Could you check a few things on this model? Use its own coordinates, in mm. Give positions to 0.01 mm unless a question says otherwise; leave off trailing zeros. Write each loop counter-clockwise with the first axis right and the second up, starting at its lowest first coordinate (ties: lowest second). Pieces come first, ordered by that corner, then holes. Notation, with made-up numbers: M -13,85 L 0,85 A32 ccw 0,115 Z; hole C 8,10 d1. An arc over 180 degrees is marked long. Use one line per item in the form item = value.
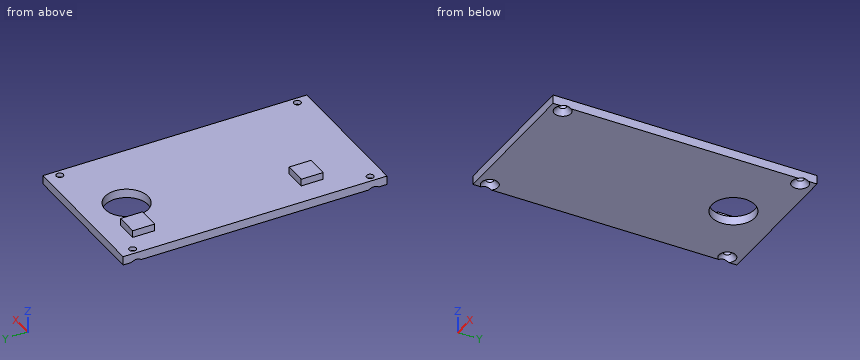
from build123d import *

# Parameters (mm, degrees)
SKETCH1_W           = 33.15
SKETCH1_H           = 60
SKETCH1_R           = 4.9
BOSS_EXTRUDE1_DEPTH = 2
SKETCH3_W           = 5
SKETCH3_H           = 5
BOSS_EXTRUDE2_DEPTH = 1.6
SKETCH4_R           = 0.8
CUT_EXTRUDE1_DEPTH  = 2
CHAMFER1_SIZE       = 1.1


with BuildPart() as part:
    # Sketch1 → Boss-Extrude1 (new body)
    with BuildSketch(Plane.XY):
        Rectangle(SKETCH1_W, SKETCH1_H)
        with Locations((0, 20.1)):
            Circle(SKETCH1_R, mode=Mode.SUBTRACT)
    extrude(amount=BOSS_EXTRUDE1_DEPTH)

    # Sketch3 → Boss-Extrude2 (add)
    with BuildSketch(Plane.XY.offset(2)):
        with Locations((-8.94, 22.5)):
            Rectangle(SKETCH3_W, SKETCH3_H)
        with Locations((-8.94, -15.82)):
            Rectangle(SKETCH3_W, SKETCH3_H)
    extrude(amount=BOSS_EXTRUDE2_DEPTH)

    # Sketch4 → Cut-Extrude1 (cut)
    with BuildSketch(Plane(origin=(0, 0, 0), x_dir=(-1, 0, 0), z_dir=(0, 0, -1))):
        with Locations((-15.075, 27)):
            Circle(SKETCH4_R)
        with Locations((15.075, 27)):
            Circle(SKETCH4_R)
        with Locations((15.075, -27)):
            Circle(SKETCH4_R)
        with Locations((-15.075, -27)):
            Circle(SKETCH4_R)
    extrude(amount=-CUT_EXTRUDE1_DEPTH, mode=Mode.SUBTRACT)

    # Chamfer1
    # the kernel refuses this chamfer: 1.1 mm, written as the material it takes off along each edge
    with BuildSketch(Plane(origin=(15.075, -27, 0), x_dir=(-1, 0, 0), z_dir=(0, -1, 0))) as chamfer1_piece_1:
        Polygon((0.8 + CHAMFER1_SIZE, 0), (0.8, -CHAMFER1_SIZE), (0.8, 0), align=None)
    revolve(axis=Axis((15.075, -27, 0), (0, 0, -1)), mode=Mode.SUBTRACT)
    with BuildSketch(Plane(origin=(-15.075, -27, 0), x_dir=(-1, 0, 0), z_dir=(0, -1, 0))) as chamfer1_piece_2:
        Polygon((0.8 + CHAMFER1_SIZE, 0), (0.8, -CHAMFER1_SIZE), (0.8, 0), align=None)
    revolve(axis=Axis((-15.075, -27, 0), (0, 0, -1)), mode=Mode.SUBTRACT)
    with BuildSketch(Plane(origin=(-15.075, 27, 0), x_dir=(-1, 0, 0), z_dir=(0, -1, 0))) as chamfer1_piece_3:
        Polygon((0.8 + CHAMFER1_SIZE, 0), (0.8, -CHAMFER1_SIZE), (0.8, 0), align=None)
    revolve(axis=Axis((-15.075, 27, 0), (0, 0, -1)), mode=Mode.SUBTRACT)
    with BuildSketch(Plane(origin=(15.075, 27, 0), x_dir=(-1, 0, 0), z_dir=(0, -1, 0))) as chamfer1_piece_4:
        Polygon((0.8 + CHAMFER1_SIZE, 0), (0.8, -CHAMFER1_SIZE), (0.8, 0), align=None)
    revolve(axis=Axis((15.075, 27, 0), (0, 0, -1)), mode=Mode.SUBTRACT)


solid = part.part
1) I want a section at B-B, the plane x = 0. Please give me the cut outline in (y, z), plus the area to 3 significant figures.
Checked values:
outline = M -30,0 L 15.2,0 L 15.2,2 L -30,2 Z; M 25,0 L 30,0 L 30,2 L 25,2 Z
area = 100 mm2
2) I want a section at A-A, the plane y = 27. Please give me the cut outline in (x, z) (3 decimals), plus the area to 3 significant figures.
Checked values:
outline = M -16.575,0.4 L -15.875,1.1 L -15.875,2 L -16.575,2 Z; M -14.275,1.1 L -13.175,0 L 13.175,0 L 14.275,1.1 L 14.275,2 L -14.275,2 Z; M 15.875,1.1 L 16.575,0.4 L 16.575,2 L 15.875,2 Z
area = 57.6 mm2
3) I want a section at C-C, the plane z = 2.65. Please give me the cut outline in (x, y).
Checked values:
outline = M -11.44,-18.32 L -6.44,-18.32 L -6.44,-13.32 L -11.44,-13.32 Z; M -11.44,20 L -6.44,20 L -6.44,25 L -11.44,25 Z
4) For pin 1 Ø1.5 at (x, y) = (4.5, 1) entering from +Z; pin 2 Ø0.8 at (x, z) = (-8, 2.5) entering from -Y; pin 3 Ø2.5 at (x, y) = (15.075, 27) entering from -Z; pin 4 Ø1.3 at (x, y) = (-15.075, 27) entering from +Z, each with a flat end and sliding along its axis, tell me the tip position at first contact or that it passes through.
Checked values:
pin_1 = 2
pin_2 = -18.32
pin_3 = 0.65
pin_4 = through
5) If I drill on L1, parallel to X at y = 20, z = 1.5 (3 decimals); L2, parallel to X at y = 18.5, z = 0.4 (3 decimals); L3, parallel to Y at x = -1.5, z = 0.2, over which ranges is the centre line in solid material (lowest first)?
Checked values:
L1 = -16.575 to -4.899, 4.899 to 16.575
L2 = -16.575 to -4.631, 4.631 to 16.575
L3 = -30 to 15.44, 24.76 to 30
6) I want a section at D-D, the plane x = -10. Please give me the cut outline in (y, z).
Checked values:
outline = M -30,0 L 30,0 L 30,2 L 25,2 L 25,3.6 L 20,3.6 L 20,2 L -13.32,2 L -13.32,3.6 L -18.32,3.6 L -18.32,2 L -30,2 Z
